Geometry: final body of the model. Coordinates: model frame, mm. Round coordinates to 2 decimals unless told otherwise and drop trailing zeros. Write each loop counter-clockwise with the first axis right and the second up, starting at its lowest first coordinate (ties: lowest second). Pieces come first, ordered by that corner, then holes. Notation, with made-up numbers: M 28.5,-27.75 L 37.5,-27.75 A20 cw 37.5,-18.75 Z; hole C 19.5,8.25 d4. An arc over 180 degrees is marked long. Use one line per item in the form item = value. Start each with the question number.
Item 1: Section query C-C (x = 530). Return loops of the section in (y, z).
Item 2: Pin query (flat end, axial travel): pin 1 Ø13 at (x, y) = (30, 220) entering from +Z; pin 2 Ø2 at (y, z) = (475, 7.5) entering from -X; pin 3 Ø6 at (y, z) = (304, 8) entering from +X. Return the tip coordinate at first contact, or that it passes through.
Item 3: Section query D-D (x = 360.5). Return loops of the section in (y, z), and give its area (3 significant figures).
Item 4: Ray query, probe 1 along X at (y, z) = (216, 7); probe 2 along Y at (x, z) = (1030, 2.75); probe 3 along X at (y, z) = (215, 7.5) (3 decimals). Return the intervals inside material, ascending.
Item 5: Section query A-A (y = 309). Return loops of the section in (x, z), and give its area (3 significant figures).
Item 6: Section query B-B (z = 7.5). Return loops of the section in (x, y), and give its area (3 significant figures).
from build123d import *

# Parameters (mm, degrees)
SKETCH_1_W                  = 1060
SKETCH_1_H                  = 530
EXTRUDE_1_DEPTH             = 10
CUT_EXTRUDE_1_DEPTH         = 10
CHAMFER_1_SIZE              = 300
HOLE_WIZARD_16_0_16_1_D     = 16
HOLE_WIZARD_16_0_16_1_DEPTH = 42
HOLE_WIZARD_16_0_16_1_TIP   = 4.806884952


with BuildPart() as part:
    # 草图1 → 凸台-拉伸1 (new body)
    with BuildSketch(Plane.XY):
        with Locations((530, 265)):
            Rectangle(SKETCH_1_W, SKETCH_1_H)
    extrude(amount=EXTRUDE_1_DEPTH)

    # 草图2 → 切除-拉伸1 (cut)
    with BuildSketch(Plane.XY.offset(10)):
        with BuildLine():
            Line((96, 20), (96, 0))
            Line((96, 0), (964, 0))
            Line((964, 0), (964, 20))
            ThreePointArc((964, 20), (530, 454), (96, 20))
        make_face()
    extrude(amount=-CUT_EXTRUDE_1_DEPTH, mode=Mode.SUBTRACT)

    # 倒角1
    chamfer_1_edges = [part.edges().sort_by_distance(p)[0] for p in [
        (0, 530, 5),
        (1060, 530, 5),
    ]]
    chamfer(chamfer_1_edges, length=CHAMFER_1_SIZE)

    # Ø16.0 (16) 直径孔1
    with Locations(Plane.XY.offset(10)):
        with Locations((30, 220), (30, 50), (1030, 220), (1030, 50), (310, 500), (750, 500)):
            Hole(HOLE_WIZARD_16_0_16_1_D / 2, depth=HOLE_WIZARD_16_0_16_1_DEPTH)
            with Locations((0, 0, -(HOLE_WIZARD_16_0_16_1_DEPTH + HOLE_WIZARD_16_0_16_1_TIP / 2))):  # 118° drill point
                Cone(0, HOLE_WIZARD_16_0_16_1_D / 2, HOLE_WIZARD_16_0_16_1_TIP, mode=Mode.SUBTRACT)


solid = part.part
Working result:
q1.outline = M 454,0 L 530,0 L 530,10 L 454,10 Z
q2.pin_1 = through
q2.pin_2 = 244
q2.pin_3 = 989
q3.outline = M 419.53,0 L 530,0 L 530,10 L 419.53,10 Z
q3.area = 1,100 mm²
q4.probe_1 = 0 to 23.07, 36.93 to 142.78, 917.22 to 1023.07, 1036.93 to 1060
q4.probe_2 = 0 to 42, 58 to 212, 228 to 260
q4.probe_3 = 0 to 23.755, 36.245 to 142.275, 917.725 to 1023.755, 1036.245 to 1060
q5.outline = M 79,0 L 206.22,0 L 206.22,10 L 79,10 Z; M 853.78,0 L 981,0 L 981,10 L 853.78,10 Z
q5.area = 2,540 mm²
q6.outline = M 0,0 L 96,0 L 96,20 A434 cw 964,20 L 964,0 L 1060,0 L 1060,230 L 760,530 L 300,530 L 0,230 Z; hole C 30,50 d16; hole C 30,220 d16; hole C 310,500 d16; hole C 750,500 d16; hole C 1030,50 d16; hole C 1030,220 d16
q6.area = 157,000 mm²
